CAD build for the part. Positions are in the model's coordinates, mm. Round coordinates to 2 decimals unless told otherwise and drop trailing zeros. Loops run counter-clockwise (first coordinate to the right, second up) from the corner with the lowest first, then second, coordinate; pieces in that order, holes last.
Solid Edge part; units mm, degrees
sketch "Sketch1" plane through (0, 0, 0) normal (0, 0, 1) x (1, 0, 0)
  line L0 (-15, -2.5) -> (15, -2.5)
  line L1 (15, -2.5) -> (15, 2.5)
  line L2 (15, 2.5) -> (-15, 2.5)
  line L3 (-15, 2.5) -> (-15, -2.5)
  dimension "D1" = 15
  dimension "D2" = 15
extrude "Protrusion1" add sketch "Sketch1" along normal blind 4.5
sketch "Sketch2" plane through (0, 0, 4.5) normal (0, 0, 1) x (1, 0, 0)
  circle A0 centre (-8.5, 0) radius 1.25
  circle A1 centre (8.5, 0) radius 1.25
extrude "Cutout1" cut sketch "Sketch2" against normal through all
properties material "ABS Plastic, medium impact"
Item 1: Two-plate mould, pull along X, no slides. Class faces 1 (the cylindrical face through (7.25, 0.05, 2.28)), 2 (the flat face through (0, 2.5, 2)), 3 (the flat face through (-15, 0, 2)), 4 (the flat face through (15, 0, 2)): released by +X, released by -X, zero draft, split by the parting line, or undercut.
Answers follow:
face 1: undercut
face 2: zero draft
face 3: released by -X
face 4: released by +X
Item 2: Cut at B-B, the plane y = 0. Give the cut face in (x, z), plus the area to 4 significant figures.
Answers follow:
outline: (-15, 0) - (-9.75, 0) - (-9.75, 4.5) - (-15, 4.5) - close; (-7.25, 0) - (7.25, 0) - (7.25, 4.5) - (-7.25, 4.5) - close; (9.75, 0) - (15, 0) - (15, 4.5) - (9.75, 4.5) - close
area: 112.5 mm2
Item 3: Cut at C-C, the plane z = 1.85. Give the cut face in (x, y), plus the area to 3 significant figures.
Answers follow:
outline: (-15, -2.5) - (15, -2.5) - (15, 2.5) - (-15, 2.5) - close; hole circle Ø2.5 at (-8.5, 0); hole circle Ø2.5 at (8.5, 0)
area: 140 mm2
Item 4: Probe line 1 (Y direction, x = 8.5, z = 1.1); line 2 (X direction, y = -1, z = 1.85); line 3 (X direction, y = -0.9, z = 0.8). List the from-to ranges inside material, lowest first.
Answers follow:
line 1: y = -2.5 to -1.25, 1.25 to 2.5
line 2: x = -15 to -9.25, -7.75 to 7.75, 9.25 to 15
line 3: x = -15 to -9.37, -7.63 to 7.63, 9.37 to 15
Item 5: Cut at A-A, the plane x = -8.5. Give the cut face in (y, z), plus the area to 4 significant figures.
Answers follow:
outline: (-2.5, 0) - (-1.25, 0) - (-1.25, 4.5) - (-2.5, 4.5) - close; (1.25, 0) - (2.5, 0) - (2.5, 4.5) - (1.25, 4.5) - close
area: 11.25 mm2
